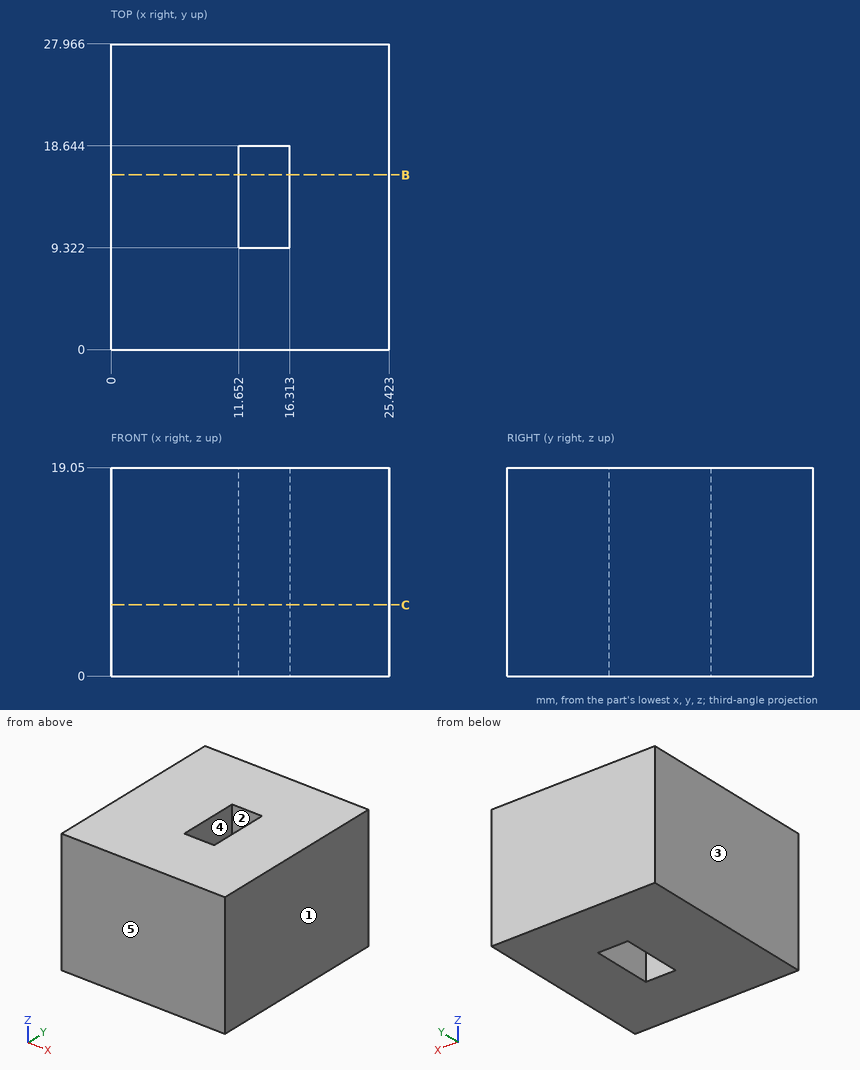
Verification items for this drawing (mm, ordinates from the low corner). A direction names the side the tool comes from. Coordinates: 2 decimals unless noted, no trailing zeros. Write each loop counter-clockwise with the first axis right and the second up, starting at its lowest first coordinate (ties: lowest second). Pieces come first, ordered by that corner, then holes. Notation, with made-up numbers: (57, 10.5) -> (116, 10.5) arc R24 ccw to (116, 21.5) -> close; hole circle Ø8 at (79.25, 79.5). An arc over 180 degrees is marked (long way). One line per item, written item: value. Start each with the question number.
Q1. Thickness scan on L1, parallel to X at y = 16, z = 5; L2, parallel to Y at x = 13.5, z = 6.75 (1 decimal). Record the ranges inside material, lowest first. Write a range as from..to.
Q2. Cross-section at B-B on y = 16. Enter the section's corners in (x, z).
Q3. Access from +Z, -Z, +X, -X, +Y, -Y to the whole of each face (thin tool, end or side, straight path). Record for the marked faces 1 and 2.
Q4. Mould release check, pull along Y, two halves, no side actions. Record for the marked faces 3, 4 and 5: pulls with the +Y half, pulls with the -Y half, needs draft (parallel to the pull), parting line crosses it, or undercut.
Q5. Cross-section at C-C on z = 6.5. Enter the section's corners in (x, y) (1 decimal).
Checked values:
1. L1: x = 0..11.65, 16.31..25.42
1. L2: y = 0..9.3, 18.6..28
2. outline: (0, 0) -> (11.65, 0) -> (11.65, 19.05) -> (0, 19.05) -> close; (16.31, 0) -> (25.42, 0) -> (25.42, 19.05) -> (16.31, 19.05) -> close
3. face 1: +Z, -Z, +X, +Y, -Y
3. face 2: +Z, -Z
4. face 3: needs draft
4. face 4: undercut
4. face 5: pulls with the -Y half
5. outline: (0, 0) -> (25.4, 0) -> (25.4, 28) -> (0, 28) -> close; hole (11.7, 9.3) -> (16.3, 9.3) -> (16.3, 18.6) -> (11.7, 18.6) -> close
